Geometry check sheet. Reference: the model listing, model coordinates, mm. A direction names the side the tool comes from. Coordinates: 2 decimals unless noted, no trailing zeros. Write each loop counter-clockwise with the first axis right and the second up, starting at its lowest first coordinate (ties: lowest second). Pieces come first, ordered by that corner, then holes. Notation, with made-up numbers: (-2, 80) -> (18, 80) arc R20 ccw to (18, 96) -> close; hole circle Ø6 at (-31.75, 29.25). An arc over 180 degrees is marked (long way). One line per question, with ' | ' between items.
```python
from build123d import *

# Parameters (mm, degrees)
SKETCH1_W                        = 203.2
SKETCH1_H                        = 228.6
CHASSIS_DEPTH                    = 76.2
CHASSIS_COMPARTMENT_T            = -12.7
OUTER_FILLETS_R                  = 10
LEFT_MOTOR_COMPARTMENTS_DEPTH    = 8.7
RIGHT_START                      = -8.7
RIGHT_MOTOR_COMPARTMENTS_DEPTH   = 8.7
SKETCH8_R                        = 4
SKETCH8_R_2                      = 3.999993352
LID_HOLES_DEPTH                  = 10
SCREW_AND_SHAFT_HOLES_DEPTH      = 278.790948922
SCREW_AND_SHAFT_HOLES_DEPTH_BACK = 278.790948922
SKETCH10_R                       = 3.25
SKETCH10_R_2                     = 6.5


with BuildPart() as part:
    # Sketch1 → Chassis (new body)
    with BuildSketch(Plane.XY):
        with Locations((-5.130884808, -63.69081803)):
            Rectangle(SKETCH1_W, SKETCH1_H)
    extrude(amount=CHASSIS_DEPTH)

    # Chassis Compartment
    chassis_compartment_openings = [part.faces().sort_by_distance(p)[0] for p in [
        (-5.130884808, -63.69081803, 76.2),
    ]]
    offset(amount=CHASSIS_COMPARTMENT_T, openings=chassis_compartment_openings, kind=Kind.INTERSECTION)

    # Outer Fillets
    outer_fillets_edges = [part.edges().sort_by_distance(p)[0] for p in [
        (-106.730884808, 50.60918197, 38.1),
        (96.469115192, 50.60918197, 38.1),
        (96.469115192, -177.99081803, 38.1),
        (-106.730884808, -177.99081803, 38.1),
    ]]
    fillet(outer_fillets_edges, radius=OUTER_FILLETS_R)

    # Sketch3 → Left Motor Compartments (cut)
    with BuildSketch(Plane.ZY.offset(94.030884808)):
        with BuildLine():
            Line((31.75, -162.09081803), (12.7, -162.09081803))
            Line((12.7, -162.09081803), (12.7, -123.99081803))
            Line((12.7, -123.99081803), (31.75, -123.99081803))
            ThreePointArc((31.75, -123.99081803), (50.8, -143.04081803), (31.75, -162.09081803))
        make_face()
        with BuildLine():
            Line((31.75, -3.39081803), (12.7, -3.39081803))
            Line((12.7, -3.39081803), (12.7, 34.70918197))
            Line((12.7, 34.70918197), (31.75, 34.70918197))
            ThreePointArc((31.75, 34.70918197), (50.8, 15.65918197), (31.75, -3.39081803))
        make_face()
    extrude(amount=LEFT_MOTOR_COMPARTMENTS_DEPTH, mode=Mode.SUBTRACT)

    # Sketch5 → Right Motor Compartments (cut)
    with BuildSketch(Plane.ZY.offset(-83.769115192).offset(RIGHT_START)):
        with BuildLine():
            Line((31.75, 34.70918197), (12.7, 34.70918197))
            Line((12.7, 34.70918197), (12.7, -3.39081803))
            Line((12.7, -3.39081803), (31.75, -3.39081803))
            ThreePointArc((31.75, -3.39081803), (50.8, 15.65918197), (31.75, 34.70918197))
        make_face()
        with BuildLine():
            Line((31.75, -123.99081803), (12.7, -123.99081803))
            Line((12.7, -123.99081803), (12.7, -162.09081803))
            Line((12.7, -162.09081803), (31.75, -162.09081803))
            ThreePointArc((31.75, -162.09081803), (50.8, -143.04081803), (31.75, -123.99081803))
        make_face()
    extrude(amount=RIGHT_MOTOR_COMPARTMENTS_DEPTH, mode=Mode.SUBTRACT)

    # Sketch8 → Lid Holes (cut)
    with BuildSketch(Plane.XY.offset(76.2)):
        with Locations((88.590435536, 42.730502314)):
            Circle(SKETCH8_R)
        with Locations((-98.836735073, 42.746020894)):
            Circle(SKETCH8_R_2)
        with Locations((88.590435536, -170.112138374)):
            Circle(SKETCH8_R_2)
        with Locations((-98.852205152, -170.112138374)):
            Circle(SKETCH8_R_2)
    extrude(amount=-LID_HOLES_DEPTH, mode=Mode.SUBTRACT)

    # Sketch10 → Screw and Shaft Holes (cut, two sides: drawn at the far end of the back side and taken through both)
    with BuildSketch(Plane(origin=(-102.730884808, 0, 0), x_dir=(0, 0, -1), z_dir=(1, 0, 0)).offset(-SCREW_AND_SHAFT_HOLES_DEPTH_BACK)):
        with Locations(Location((-31.75, -127.54081803, 0), (0, 0, 90))):
            Circle(SKETCH10_R)
        with Locations(Location((-45.173393759, -135.29081803, 0), (0, 0, 90))):
            Circle(SKETCH10_R)
        with Locations(Location((-18.326606241, -135.29081803, 0), (0, 0, 90))):
            Circle(SKETCH10_R)
        with Locations(Location((-45.173393759, -150.79081803, 0), (0, 0, 90))):
            Circle(SKETCH10_R)
        with Locations(Location((-18.326606241, -150.79081803, 0), (0, 0, 90))):
            Circle(SKETCH10_R)
        with Locations(Location((-31.75, -158.54081803, 0), (0, 0, 90))):
            Circle(SKETCH10_R)
        with Locations(Location((-31.75, 31.15918197, 0), (0, 0, 90))):
            Circle(SKETCH10_R)
        with Locations(Location((-45.173393759, 23.40918197, 0), (0, 0, 90))):
            Circle(SKETCH10_R)
        with Locations(Location((-18.326606241, 23.40918197, 0), (0, 0, 90))):
            Circle(SKETCH10_R)
        with Locations(Location((-45.173393759, 7.90918197, 0), (0, 0, 90))):
            Circle(SKETCH10_R)
        with Locations(Location((-18.326606241, 7.90918197, 0), (0, 0, 90))):
            Circle(SKETCH10_R)
        with Locations(Location((-31.75, 0.15918197, 0), (0, 0, 90))):
            Circle(SKETCH10_R)
        with Locations(Location((-24.75, -143.04081803, 0), (0, 0, 90))):
            Circle(SKETCH10_R_2)
        with Locations(Location((-24.75, 15.65918197, 0), (0, 0, 90))):
            Circle(SKETCH10_R_2)
    extrude(amount=SCREW_AND_SHAFT_HOLES_DEPTH + SCREW_AND_SHAFT_HOLES_DEPTH_BACK, mode=Mode.SUBTRACT)


solid = part.part
```
(1) Cross-section at B-B (y = -20). Record the cut outline in (x, z).
Answers below:
outline: (-106.73, 0) -> (96.47, 0) -> (96.47, 76.2) -> (83.77, 76.2) -> (83.77, 12.7) -> (-94.03, 12.7) -> (-94.03, 76.2) -> (-106.73, 76.2) -> close
(2) Cross-section at A-A (z = 61.5). Record the cut outline in (x, y), plus the area to 3 significant figures.
Answers below:
outline: (-106.73, -167.99) arc R10 ccw to (-96.73, -177.99) -> (86.47, -177.99) arc R10 ccw to (96.47, -167.99) -> (96.47, 40.61) arc R10 ccw to (86.47, 50.61) -> (-96.73, 50.61) arc R10 ccw to (-106.73, 40.61) -> close; hole (-94.03, -165.29) -> (83.77, -165.29) -> (83.77, 37.91) -> (-94.03, 37.91) -> close | area: 10,200 mm²
(3) Cross-section at D-D (z = 24.75). Count the separate pieces of the cut face and the enclosed holes in it, plus the area to 3 significant figures.
Answers below:
separate pieces: 4 | enclosed holes: 0 | area: 8,700 mm²
(4) Draft check along Z on faces 4 (the face through (89, 43, 66.2)), 5 (the face through (-6, -177.991, 38)), 6 (the face through (-104.76, -132.19, 19.3)). Enter one of: pulls with the +Z half, pulls with the -Z half, needs draft (parallel to the pull), parting line crosses it, or undercut.
Answers below:
face 4: pulls with the +Z half | face 5: needs draft | face 6: undercut
(5) Cross-section at C-C (x = -20). Record the cut outline in (y, z), plus the area to 3 significant figures.
Answers below:
outline: (-177.99, 0) -> (50.61, 0) -> (50.61, 76.2) -> (37.91, 76.2) -> (37.91, 12.7) -> (-165.29, 12.7) -> (-165.29, 76.2) -> (-177.99, 76.2) -> close | area: 4,520 mm²
(6) Depth check by flat-ended pin: P1, Ø4, axis at x = 89.5, y = -171.5, coming from the +Z side; P2, Ø12, axis at x = -67.5, y = -96, coming from the +Z side. Enter the tip coordinate at first touch or a pass-through.
Answers below:
P1: stops at z = 66.2 | P2: stops at z = 12.7
(7) Tool access check on faces 1 (the face through (-98.32, 16.078, 50.795)), 2 (the face through (-94.031, -65, 51)), 3 (the face through (-103.88, 47.6, 38.63)). Record the directions out of +Z, -Z, +X, -X, +Y, -Y that give a thin tool (end or side, any length) a straight path to the whole face; none if there is none.
Answers below:
face 1: none | face 2: +Z | face 3: +Z, -Z, -X, +Y
(8) Material ranges on line 1 (Y direction, x = 85.5, z = 35); line 2 (X direction, y = 9.5, z = 35); line 3 (Y direction, x = 65, z = 65.5), recorded low to high.
Answers below:
line 1: y = -177.99 to -161.81, -124.27 to -3.11, 34.43 to 50.61 | line 2: x = -106.73 to -102.73, 92.47 to 96.47 | line 3: y = -177.99 to -165.29, 37.91 to 50.61
